Work out the finished part from the listing and answer in its coordinate system (mm). A direction names the side the tool comes from. Coordinates: 2 decimals unless noted, no trailing zeros. Order: outer loops, then holes, each group sorted by start corner. A loop starts at its lowest first (then second) coordinate and runs counter-clockwise, first axis right, second up. Notation, with made-up numbers: M -35.75,52.25 L 5.25,52.25 A9 cw 5.25,57.25 Z; hole C -7.5,80 d1. An arc over 180 degrees is marked long. Answer in a Markdown table with one row per item. Add a question column.
Item 1: Consider line 1 (Y direction, x = 24.5, z = 0); line 2 (X direction, y = -3.5, z = 2.5); line 3 (Z direction, x = -30.25, y = -7.5). Determine where each line is inside the solid, lowest interval first. Write a range as from..to.
Item 2: The mould has two halves that part along X. Classify faces 1 (the face through (13.254, -7.395, 0.176)), 2 (the face through (-2, -15, 0)), 3 (the face through (-33.25, -9.1, -2.4)): released by +X, released by -X, zero draft, split by the parting line, or undercut.
Item 3: The part is cut by section A-A (x = -19.25). Write down the section's boundary in (y, z), then the cut area to 3 significant figures.
Item 4: Which of the six approach directions +Z, -Z, +X, -X, +Y, -Y give full straight-line access (tool end or side, diameter ignored) to faces 4 (the face through (-29.834, -9.885, 0.751)), 5 (the face through (24.87, -7.83, 2.48)), 6 (the face through (29.25, -9.1, -2.4))?
Item 5: The part is cut by section C-C (x = 24). Write down the section's boundary in (y, z).
Item 6: The part is cut by section B-B (z = 0). Write down the section's boundary in (x, y).
Item 7: The part is cut by section D-D (y = -12). Write down the section's boundary in (x, z), then the cut area to 3 significant figures.
Item 8: Flat-ended cylindrical pins translate along their axes: pin 1 Ø4.5 at (y, z) = (-7.5, 0) entering from -X; pin 2 Ø1 at (y, z) = (-8.5, 1.5) entering from +X; pin 3 Ø5 at (x, z) = (17.25, 0) entering from +Y. Find the tip coordinate at first contact, or state that the pin passes through.
from build123d import *

# Parameters (mm, degrees)
F0_W        = 62.5
F0_H        = 20
F0_R        = 7.5
F0_R_2      = 4
F1_DEPTH    = 7.5
F1_FACE_W   = 62.5
F1_FACE_H   = 20
F1_FACE_R   = 7.5
F1_FACE_R_2 = 4
F2_DEPTH    = 7.5
F3_R        = 2.5
F4_DEPTH    = 10
F5_R        = 2.5
F6_DEPTH    = 12


with BuildPart() as f1:
    # F0 (on Front) → F1 (new body)
    with BuildSketch(Plane.XZ):
        with Locations((-2, 0)):
            Rectangle(F0_W, F0_H)
        with Locations((-19.25, 0)):
            Circle(F0_R, mode=Mode.SUBTRACT)
        with Locations((17.25, 0)):
            Circle(F0_R_2, mode=Mode.SUBTRACT)
    extrude(amount=F1_DEPTH)

    # F1_face (on face) → F2 (join)
    with BuildSketch(Plane(origin=(0.033896, -7.5, 0), x_dir=(1, 0, 0), z_dir=(0, -1, 0))):
        with Locations((-2.033896, 0)):
            Rectangle(F1_FACE_W, F1_FACE_H)
        with Locations((-19.283896, 0)):
            Circle(F1_FACE_R, mode=Mode.SUBTRACT)
        with Locations((17.216104, 0)):
            Circle(F1_FACE_R_2, mode=Mode.SUBTRACT)
    extrude(amount=F2_DEPTH)

    # F3 (on face) → F4 (cut)
    with BuildSketch(Plane(origin=(-33.25, 0, 0), x_dir=(0, -1, 0), z_dir=(-1, 0, 0))):
        with Locations((7.5, 0)):
            Circle(F3_R)
    extrude(amount=-F4_DEPTH, mode=Mode.SUBTRACT)

    # F5 (on face) → F6 (cut)
    with BuildSketch(Plane.YZ.offset(29.25)):
        with Locations((-7.5, 0)):
            Circle(F5_R)
    extrude(amount=-F6_DEPTH, mode=Mode.SUBTRACT)


solid = f1.part
Reply:
| question | item | result |
|---|---|---|
| 1 | line 1 | y = -15..-10, -5..0 |
| 1 | line 2 | x = -33.25..-26.32, -12.18..14.13, 20.37..29.25 |
| 1 | line 3 | z = -10..-2.5, 2.5..10 |
| 2 | face 1 | undercut |
| 2 | face 2 | zero draft |
| 2 | face 3 | released by -X |
| 3 | outline | M -15,-10 L 0,-10 L 0,-7.5 L -15,-7.5 Z; M -15,7.5 L 0,7.5 L 0,10 L -15,10 Z |
| 3 | area | 75.0 mm2 |
| 4 | face 4 | -X |
| 4 | face 5 | +X |
| 4 | face 6 | +Z, -Z, +X, +Y, -Y |
| 5 | outline | M -15,-10 L 0,-10 L 0,10 L -15,10 Z; hole C -7.5,0 d5 |
| 6 | outline | M -33.25,-15 L -26.75,-15 L -26.75,-10 L -33.25,-10 Z; M -33.25,-5 L -26.75,-5 L -26.75,0 L -33.25,0 Z; M -11.75,-15 L 13.25,-15 L 13.25,0 L -11.75,0 Z; M 21.25,-15 L 29.25,-15 L 29.25,-10 L 21.25,-10 Z; M 21.25,-5 L 29.25,-5 L 29.25,0 L 21.25,0 Z |
| 7 | outline | M -33.25,-10 L 29.25,-10 L 29.25,10 L -33.25,10 Z; hole C -19.25,0 d15; hole C 17.25,0 d8 |
| 7 | area | 1,020 mm2 |
| 8 | pin 1 | stops at x = -12.1 |
| 8 | pin 2 | stops at x = 13.79 |
| 8 | pin 3 | passes through |
